Study the drawing (mm; zero at the part's minimum x, y, z) and answer. A direction names the side the tool comes from. Coordinates: 2 decimals unless noted, no trailing zeros. Order: outer loops, then holes, each group sorted by start corner. A loop starts at its lowest first (then second) coordinate and runs counter-clockwise, first axis right, second up. Notation, with made-up numbers: (12.5, 86.5) -> (20.5, 86.5) arc R27 ccw to (20.5, 124.5) -> close; hole circle Ø7 at (-3, -15.5). An arc over 180 degrees is marked (long way). Answer as CSV lines item,"result". Start each with the question number.
Item 1: Straight lines are drawn through the part: L1, parallel to Y at x = 12.5, z = 37; L2, parallel to Z at x = 13.25, y = 12.75; L3, parallel to Z at x = 11.5, y = 13.75 (1 decimal). For each, find the intervals that lie inside material, in ascending order.
Item 2: Section B-B (z = 37) is taken. Write down the section's boundary in (x, y).
Item 3: Each of these flat-tipped pins is pushed along its axis until it touches: pin 1 Ø1.5 at (y, z) = (6.5, 18.5) entering from +X; pin 2 Ø4 at (x, y) = (14.5, 10.5) entering from +Z; pin 3 Ø10 at (x, y) = (16.5, 7.5) entering from -Z. Where does it stop, or does it pass through?
Item 4: Which of the six approach directions +Z, -Z, +X, -X, +Y, -Y give full straight-line access (tool end or side, diameter ignored) to the marked faces 1, 2 and 3?
Item 5: Section D-D (z = 23) is taken. Write down the section's boundary in (x, y).
Item 6: Section A-A (x = 12.5) is taken. Write down the section's boundary in (y, z), then the cut area to 3 significant figures.
Item 7: Section C-C (y = 15.25) is taken. Write down the section's boundary in (x, z) (1 decimal).
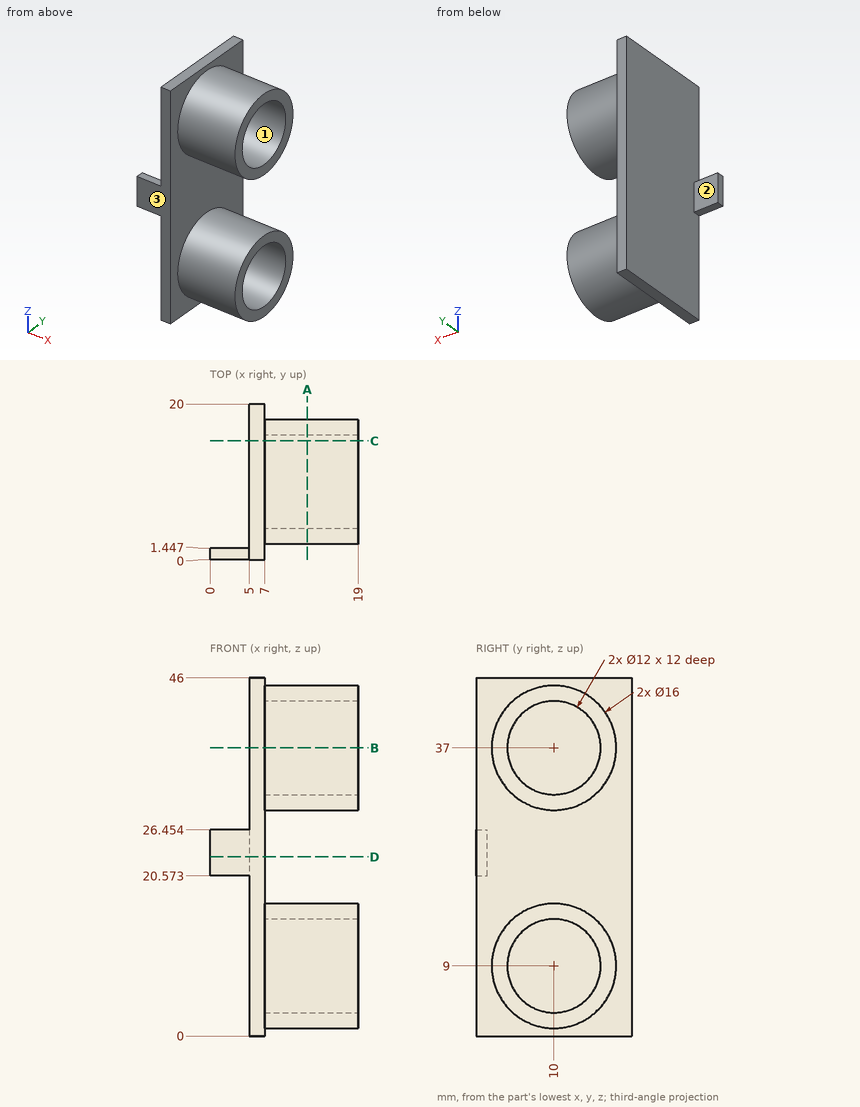
Checked values:
1,L1,"y = 2 to 4, 16 to 18"
1,L2,"z = 1.49 to 3.67, 14.33 to 16.51, 29.49 to 31.67, 42.33 to 44.51"
1,L3,"z = 1.9 to 4.3, 13.7 to 16.1, 29.9 to 32.3, 41.7 to 44.1"
2,outline,"(5, 0) -> (7, 0) -> (7, 2) -> (19, 2) -> (19, 4) -> (7, 4) -> (7, 16) -> (19, 16) -> (19, 18) -> (7, 18) -> (7, 20) -> (5, 20) -> close"
3,pin 1,"stops at x = 7"
3,pin 2,"stops at z = 45"
3,pin 3,"stops at z = 1"
4,face 1,"+X"
4,face 2,"+Z, -Z, -X, +Y"
4,face 3,"+Z, -Z, +X, -X, -Y"
5,outline,"(0, 0) -> (7, 0) -> (7, 20) -> (5, 20) -> (5, 1.45) -> (0, 1.45) -> close"
6,outline,"circle Ø16 at (10, 9); circle Ø16 at (10, 37); hole circle Ø12 at (10, 9); hole circle Ø12 at (10, 37)"
6,area,"176 mm^2"
7,outline,"(5, 0) -> (7, 0) -> (7, 3) -> (19, 3) -> (19, 6.1) -> (7, 6.1) -> (7, 11.9) -> (19, 11.9) -> (19, 15) -> (7, 15) -> (7, 31) -> (19, 31) -> (19, 34.1) -> (7, 34.1) -> (7, 39.9) -> (19, 39.9) -> (19, 43) -> (7, 43) -> (7, 46) -> (5, 46) -> close"
